Geometry check sheet. Reference: the model listing, model coordinates, mm. A direction names the side the tool comes from. Coordinates: 2 decimals unless noted, no trailing zeros. Write each loop counter-clockwise with the first axis right and the second up, starting at its lowest first coordinate (ties: lowest second). Pieces come first, ordered by that corner, then holes. Notation, with made-up numbers: (-38, -23) -> (11, -23) arc R13 ccw to (11, -5) -> close; hole circle Ø9 at (-29.5, 78). An arc over 180 degrees is marked (long way). Answer in a Markdown table with one row per item. Add a question column.
1. Scan lines: L1, parallel to Z at x = -1.5, y = -925; L2, parallel to Y at x = -2.5, z = -9 (3 decimals); L3, parallel to X at y = -657.5, z = 5.5. Record each from-to range of solid material in increasing order. Write a range as from..to.
2. Cross-section at C-C on z = -8. Record the cut outline in (x, y) (3 decimals), and give its area (3 significant figures).
3. Cross-section at A-A on x = 0. Record the cut outline in (y, z) (3 decimals).
4. Set-up check for faces 4 (the flat face through (0, -3.175, 0)), 5 (the flat face through (0, -0.635, 0)), 6 (the flat face through (-21, 0, 10)): record each of +Z, -Z, +X, -X, +Y, -Y from which the full face is reachable in a straight line by a thin tool's end or side.
5. Mould release check, pull along Z, two halves, no side actions. Record for faces 1 (the cylindrical face through (24.23, -500.89, 7.63)), 2 (the cylindrical face through (21.2, -502.5, 6.68)), 3 (the flat face through (-0.1, -1016, -22.5)): pulls with the +Z half, pulls with the -Z half, needs draft (parallel to the pull), parting line crosses it, or undercut.
6. Cross-section at B-B on y = -579.5. Record the cut outline in (x, z).
7. Depth check by flat-ended pin: P1, Ø22, axis at x = -6, z = 6, coming from the -Y side (3 decimals); P2, Ø4, axis at x = 17.5, z = -7.5, coming from the +Y side (3 decimals); P3, Ø8, axis at x = 7.5, y = -526.5, coming from the -Z side. Enter the tip coordinate at first touch or a pass-through.
```python
from build123d import *

# Parameters (mm, degrees)
F0_R     = 25.4032998263
F1_DEPTH = 1016
F2_T     = -3.175
F3_T     = -2.54


with BuildPart() as f1:
    # F0 (on Front) → F1 (new body)
    with BuildSketch(Plane.XZ):
        Circle(F0_R)
    extrude(amount=F1_DEPTH)

    # F2
    f2_openings = [f1.faces().sort_by_distance(p)[0] for p in [
        (0, -1016, 0),
    ]]
    offset(amount=F2_T, openings=f2_openings)

    # F3
    f3_openings = [f1.faces().sort_by_distance(p)[0] for p in [
        (0, 0, 0),
    ]]
    offset(amount=F3_T, openings=f3_openings, kind=Kind.INTERSECTION)


solid = f1.part
```
Results found:
| question | item | result |
|---|---|---|
| 1 | L1 | z = -25.36..-22.18, 22.18..25.36 |
| 1 | L2 | y = -3.175..-0.635 |
| 1 | L3 | x = -24.8..-21.54, 21.54..24.8 |
| 2 | outline | (-24.111, -1016) -> (-20.739, -1016) -> (-20.739, -3.175) -> (20.739, -3.175) -> (20.739, -1016) -> (24.111, -1016) -> (24.111, 0) -> (21.418, 0) -> (21.418, -0.635) -> (-21.418, -0.635) -> (-21.418, 0) -> (-24.111, 0) -> close |
| 2 | area | 6,960 mm^2 |
| 3 | outline | (-1016, -25.403) -> (0, -25.403) -> (0, -22.863) -> (-0.635, -22.863) -> (-0.635, 22.863) -> (0, 22.863) -> (0, 25.403) -> (-1016, 25.403) -> (-1016, 22.228) -> (-3.175, 22.228) -> (-3.175, -22.228) -> (-1016, -22.228) -> close |
| 4 | face 4 | -Y |
| 4 | face 5 | +Y |
| 4 | face 6 | +Z, -Z, +X, -X, +Y |
| 5 | face 1 | parting line crosses it |
| 5 | face 2 | undercut |
| 5 | face 3 | needs draft |
| 6 | outline | circle Ø50.81 at (0, 0); hole circle Ø44.46 at (0, 0) |
| 7 | P1 | stops at y = -3.175 |
| 7 | P2 | stops at y = -0.635 |
| 7 | P3 | stops at z = -25.16 |
